CAD build for the part. Positions are in the model's coordinates, mm. A direction names the side the tool comes from. Give positions to 0.01 mm unless a question says otherwise; leave off trailing zeros. Write each loop counter-clockwise with the first axis right and the second up, starting at its lowest first coordinate (ties: lowest second). Pieces come first, ordered by that corner, then holes. Notation, with made-up numbers: (-2, 42) -> (24, 42) arc R12 cw to (24, 58) -> close; hole circle Ø2 at (3.5, 65). An arc over 180 degrees is marked (long way). Use one line per item in the form item = value. Start each with the question number.
from build123d import *

# Parameters (mm, degrees)
SKETCH1_W           = 109.982
SKETCH1_H           = 109.982
BOSS_EXTRUDE1_DEPTH = 9.0297
FILLET1_R           = 12.7
SHELL1_T            = -2.54
SKETCH2_R           = 52.07
SKETCH2_R_2         = 2.667
CUT_EXTRUDE1_DEPTH  = 79.291478745


with BuildPart() as part:
    # Sketch1 → Boss-Extrude1 (new body)
    with BuildSketch(Plane.XY):
        Rectangle(SKETCH1_W, SKETCH1_H)
    extrude(amount=BOSS_EXTRUDE1_DEPTH)

    # Fillet1
    fillet1_edges = [part.edges().sort_by_distance(p)[0] for p in [
        (54.991, -54.991, 4.51485),
        (-54.991, -54.991, 4.51485),
        (-54.991, 54.991, 4.51485),
        (54.991, 54.991, 4.51485),
    ]]
    fillet(fillet1_edges, radius=FILLET1_R)

    # Shell1
    shell1_openings = [part.faces().sort_by_distance(p)[0] for p in [
        (0, 0, 0),
    ]]
    offset(amount=SHELL1_T, openings=shell1_openings, kind=Kind.INTERSECTION)

    # Sketch2 → Cut-Extrude1 (cut, through all)
    with BuildSketch(Plane.XY.offset(9.0297)):
        Circle(SKETCH2_R)
        with Locations((43.688, 43.688)):
            Circle(SKETCH2_R_2)
        with Locations((-43.688, 43.688)):
            Circle(SKETCH2_R_2)
        with Locations((-43.688, -43.688)):
            Circle(SKETCH2_R_2)
        with Locations((43.688, -43.688)):
            Circle(SKETCH2_R_2)
    extrude(amount=-CUT_EXTRUDE1_DEPTH, mode=Mode.SUBTRACT)


solid = part.part
1) Cut at D-D (x = -44). Give the cut face in (y, z).
2) Cut at C-C (z = 2.5). Give the cut face in (x, y), and give its area (3 significant figures).
3) Wall check: line 1 along X through (y, z) = (6, 5.75); line 2 along X through (y, z) = (-0.5, 8). Give the ranges that are in metal, low to high. Write a range as from..to.
4) Cut at A-A (y = 0). Give the cut face in (x, z), and give its area (3 significant figures).
5) 3-axis set-ups, long thin cutter, end or side, ignore diameter. For faces 1 (the face through (-6.778, 51.627, 7.777)), 2 (the face through (-1, 52.451, 3)): which of +Z, -Z, +X, -X, +Y, -Y reach the whole face in a straight line?
6) Two-plate mould, pull along Y, no slides. Class faces 3 (the face through (51.17, -51.37, 4.58)), 4 (the face through (49.55, 49.4, 3.29)), 5 (the face through (51.37, 51.17, 4.58)): released by +Y, released by -Y, zero draft, split by the parting line, or undercut.
Final values:
q1.outline = (-54.88, 0) -> (-52.31, 0) -> (-52.31, 6.49) -> (-46.34, 6.49) -> (-46.34, 9.03) -> (-54.88, 9.03) -> close; (-41.04, 6.49) -> (-27.84, 6.49) -> (-27.84, 9.03) -> (-41.04, 9.03) -> close; (27.84, 6.49) -> (41.04, 6.49) -> (41.04, 9.03) -> (27.84, 9.03) -> close; (46.34, 6.49) -> (52.31, 6.49) -> (52.31, 0) -> (54.88, 0) -> (54.88, 9.03) -> (46.34, 9.03) -> close
q2.outline = (-54.99, -42.29) arc R12.7 ccw to (-42.29, -54.99) -> (42.29, -54.99) arc R12.7 ccw to (54.99, -42.29) -> (54.99, 42.29) arc R12.7 ccw to (42.29, 54.99) -> (-42.29, 54.99) arc R12.7 ccw to (-54.99, 42.29) -> close; hole (-52.45, -42.29) arc R10.16 ccw to (-42.29, -52.45) -> (42.29, -52.45) arc R10.16 ccw to (52.45, -42.29) -> (52.45, 42.29) arc R10.16 ccw to (42.29, 52.45) -> (-42.29, 52.45) arc R10.16 ccw to (-52.45, 42.29) -> close
q2.area = 1,040 mm^2
q3.line_1 = -54.99..-52.45, 52.45..54.99
q3.line_2 = -54.99..-52.07, 52.07..54.99
q4.outline = (-54.99, 0) -> (-52.45, 0) -> (-52.45, 6.49) -> (-52.07, 6.49) -> (-52.07, 9.03) -> (-54.99, 9.03) -> close; (52.07, 6.49) -> (52.45, 6.49) -> (52.45, 0) -> (54.99, 0) -> (54.99, 9.03) -> (52.07, 9.03) -> close
q4.area = 47.8 mm^2
q5.face_1 = +Z, -Z
q5.face_2 = -Z
q6.face_3 = released by -Y
q6.face_4 = undercut
q6.face_5 = released by +Y
